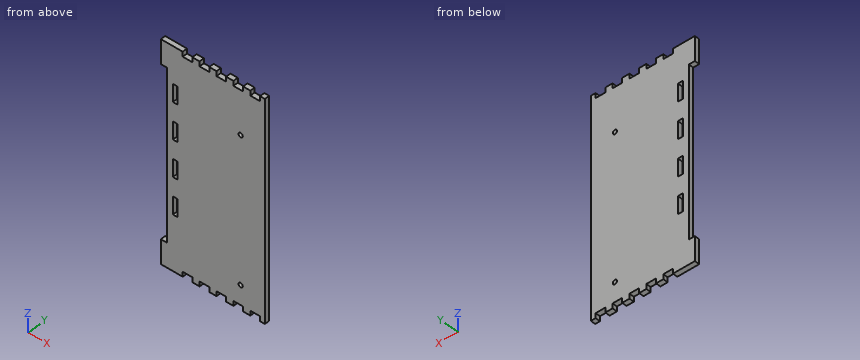
Autodesk Inventor part; units mm, degrees
ref_plane "YZ Plane" through (0, 0, 0) normal (1, 0, 0) x (0, 1, 0)
ref_plane "XZ Plane" through (0, 0, 0) normal (0, 1, 0) x (-1, 0, 0)
ref_plane "XY Plane" through (0, 0, 0) normal (0, 0, 1) x (1, 0, 0)
sketch "Sketch1" plane through (0, 0, 0) normal (0, 1, 0) x (-1, 0, 0)
  line L0 (-9.6671, 163.8128) -> (70.4329, 163.8128)
  line L1 (70.4329, 163.8128) -> (70.4329, -16.1872)
  line L2 (70.4329, -16.1872) -> (-9.6671, -16.1872)
  line L3 (-9.6671, -16.1872) -> (-9.6671, 163.8128)
  point P0 (0, 0)
extrude "Extrusion1" add sketch "Sketch1" along normal blind 4
sketch "Sketch2" plane through (0, 4, 0) normal (0, 1, 0) x (1, 0, 0)
  line L0 (-66.4329, -159.8128) -> (-66.4329, -148.8128)
  line L1 (-70.4329, -159.8128) -> (-70.4329, -148.8128)
  line L2 (-66.4329, -159.8128) -> (-66.4329, -148.8128)
  line L3 (-70.4329, -159.8128) -> (-70.4329, -148.8128)
  line L4 (-66.4329, -159.8128) -> (-66.4329, -148.8128)
  line L5 (-70.4329, -159.8128) -> (-70.4329, -148.8128)
  line L6 (-66.4329, -159.8128) -> (-66.4329, -148.8128)
  line L7 (-70.4329, -159.8128) -> (-70.4329, -148.8128)
  line L8 (-66.4329, -159.8128) -> (-66.4329, -148.8128)
  line L9 (-70.4329, -159.8128) -> (-70.4329, -148.8128)
  line L10 (-66.4329, -159.8128) -> (-66.4329, -148.8128)
  line L11 (-70.4329, -159.8128) -> (-70.4329, -148.8128)
  line L12 (-70.4329, -163.8128) -> (9.6671, -163.8128)
  line L13 (-30.3829, -163.8128) -> (-30.3829, 16.1872) construction
  line L14 (9.6671, 16.1872) -> (-70.4329, 16.1872)
  line L15 (-70.4329, -149.0628) -> (-66.4329, -149.0628)
  line L16 (-66.4329, -159.5628) -> (-70.4329, -159.5628)
  line L17 (-70.4329, 0.9372) -> (-66.4329, 0.9372)
  line L18 (-66.4329, -13.5628) -> (-70.4329, -13.5628)
  line L19 (-66.4329, -43.5628) -> (-70.4329, -43.5628)
  line L20 (-70.4329, -29.0628) -> (-66.4329, -29.0628)
  line L21 (-66.4329, -73.5628) -> (-70.4329, -73.5628)
  line L22 (-70.4329, -59.0628) -> (-66.4329, -59.0628)
  line L23 (-66.4329, -103.5628) -> (-70.4329, -103.5628)
  line L24 (-70.4329, -89.0628) -> (-66.4329, -89.0628)
  line L25 (-66.4329, -133.5628) -> (-70.4329, -133.5628)
  line L26 (-70.4329, -119.0628) -> (-66.4329, -119.0628)
  line L27 (5.6671, -159.8128) -> (5.6671, -148.8128)
  line L28 (9.6671, -159.8128) -> (9.6671, -148.8128)
  line L29 (5.6671, -133.8128) -> (5.6671, -118.8128)
  line L30 (9.6671, -133.8128) -> (9.6671, -118.8128)
  line L31 (5.6671, -103.8128) -> (5.6671, -88.8128)
  line L32 (9.6671, -103.8128) -> (9.6671, -88.8128)
  line L33 (5.6671, -73.8128) -> (5.6671, -58.8128)
  line L34 (9.6671, -73.8128) -> (9.6671, -58.8128)
  line L35 (5.6671, -43.8128) -> (5.6671, -28.8128)
  line L36 (9.6671, -43.8128) -> (9.6671, -28.8128)
  line L37 (5.6671, -13.8128) -> (5.6671, 1.1872)
  line L38 (9.6671, -13.8128) -> (9.6671, 1.1872)
  line L39 (9.6671, -149.0628) -> (5.6671, -149.0628)
  line L40 (5.6671, -159.5628) -> (9.6671, -159.5628)
  line L41 (9.6671, 0.9372) -> (5.6671, 0.9372)
  line L42 (5.6671, -13.5628) -> (9.6671, -13.5628)
  line L43 (5.6671, -43.5628) -> (9.6671, -43.5628)
  line L44 (9.6671, -29.0628) -> (5.6671, -29.0628)
  line L45 (5.6671, -73.5628) -> (9.6671, -73.5628)
  line L46 (9.6671, -59.0628) -> (5.6671, -59.0628)
  line L47 (5.6671, -103.5628) -> (9.6671, -103.5628)
  line L48 (9.6671, -89.0628) -> (5.6671, -89.0628)
  line L49 (5.6671, -133.5628) -> (9.6671, -133.5628)
  line L50 (9.6671, -119.0628) -> (5.6671, -119.0628)
  line L51 (-66.4329, -148.8128) -> (-70.4329, -148.8128)
  line L52 (-66.4329, -159.8128) -> (-70.4329, -159.8128)
  line L53 (-66.4329, -148.8128) -> (-70.4329, -148.8128)
  line L54 (-66.4329, -159.8128) -> (-70.4329, -159.8128)
  line L55 (-66.4329, -148.8128) -> (-70.4329, -148.8128)
  line L56 (-66.4329, -159.8128) -> (-70.4329, -159.8128)
  line L57 (-66.4329, -148.8128) -> (-70.4329, -148.8128)
  line L58 (-66.4329, -159.8128) -> (-70.4329, -159.8128)
  line L59 (-66.4329, -148.8128) -> (-70.4329, -148.8128)
  line L60 (-66.4329, -159.8128) -> (-70.4329, -159.8128)
  line L61 (-66.4329, -148.8128) -> (-70.4329, -148.8128)
  line L62 (-66.4329, -159.8128) -> (-70.4329, -159.8128)
  line L63 (-66.4329, -133.5628) -> (-66.4329, -119.0628)
  line L64 (-66.4329, -103.5628) -> (-66.4329, -89.0628)
  line L65 (-66.4329, -73.5628) -> (-66.4329, -59.0628)
  line L66 (-66.4329, -43.5628) -> (-66.4329, -29.0628)
  line L67 (-66.4329, -13.5628) -> (-66.4329, 0.9372)
  line L68 (-70.4329, 16.1872) -> (-70.4329, -163.8128)
  line L69 (9.6671, -163.8128) -> (9.6671, 16.1872)
  line L70 (1.6671, 16.1872) -> (1.6671, 12.1872)
  line L71 (1.6671, 12.1872) -> (-6.3329, 12.1872)
  line L72 (-6.3329, 12.1872) -> (-6.3329, 16.1872)
  line L73 (-12.3329, 16.1872) -> (-12.3329, 12.1872)
  line L74 (-12.3329, 12.1872) -> (-20.3329, 12.1872)
  line L75 (-20.3329, 12.1872) -> (-20.3329, 16.1872)
  line L76 (-26.3329, 16.1872) -> (-26.3329, 12.1872)
  line L77 (-26.3329, 12.1872) -> (-34.3329, 12.1872)
  line L78 (-34.3329, 12.1872) -> (-34.3329, 16.1872)
  line L79 (-40.3329, 16.1872) -> (-40.3329, 12.1872)
  line L80 (-40.3329, 12.1872) -> (-48.3329, 12.1872)
  line L81 (-48.3329, 12.1872) -> (-48.3329, 16.1872)
  line L82 (-54.3329, 16.1872) -> (-54.3329, 12.1872)
  line L83 (-54.3329, 12.1872) -> (-62.3329, 12.1872)
  line L84 (-62.3329, 12.1872) -> (-62.3329, 16.1872)
  line L85 (-12.3329, -73.8128) -> (-48.4329, -73.8128) construction
  line L86 (1.6671, -163.8128) -> (1.6671, -159.8128)
  line L87 (1.6671, -159.8128) -> (-6.3329, -159.8128)
  line L88 (-6.3329, -159.8128) -> (-6.3329, -163.8128)
  line L89 (-12.3329, -163.8128) -> (-12.3329, -159.8128)
  line L90 (-12.3329, -159.8128) -> (-20.3329, -159.8128)
  line L91 (-20.3329, -159.8128) -> (-20.3329, -163.8128)
  line L92 (-26.3329, -163.8128) -> (-26.3329, -159.8128)
  line L93 (-26.3329, -159.8128) -> (-34.3329, -159.8128)
  line L94 (-34.3329, -159.8128) -> (-34.3329, -163.8128)
  line L95 (-40.3329, -163.8128) -> (-40.3329, -159.8128)
  line L96 (-40.3329, -159.8128) -> (-48.3329, -159.8128)
  line L97 (-48.3329, -159.8128) -> (-48.3329, -163.8128)
  line L98 (-54.3329, -163.8128) -> (-54.3329, -159.8128)
  line L99 (-54.3329, -159.8128) -> (-62.3329, -159.8128)
  line L100 (-62.3329, -159.8128) -> (-62.3329, -163.8128)
  line L101 (9.6671, 1.1872) -> (5.6671, 1.1872)
  line L102 (9.6671, -13.8128) -> (5.6671, -13.8128)
  line L103 (9.6671, -28.8128) -> (5.6671, -28.8128)
  line L104 (9.6671, -43.8128) -> (5.6671, -43.8128)
  line L105 (9.6671, -58.8128) -> (5.6671, -58.8128)
  line L106 (5.6671, -73.8128) -> (9.6671, -73.8128)
  line L107 (9.6671, -88.8128) -> (5.6671, -88.8128)
  line L108 (9.6671, -103.8128) -> (5.6671, -103.8128)
  line L109 (9.6671, -118.8128) -> (5.6671, -118.8128)
  line L110 (9.6671, -133.8128) -> (5.6671, -133.8128)
  line L111 (9.6671, -148.8128) -> (5.6671, -148.8128)
  line L112 (9.6671, -159.8128) -> (5.6671, -159.8128)
  circle A0 centre (-14.3329, -3.8128) radius 1.75
  circle A1 centre (-14.3329, -123.8128) radius 1.75
  line L113 (5.6671, -163.8128) -> (5.6671, 16.1872)
  point P0 (0, 0)
  point P1 (-30.3829, -73.8128)
  point P2 (5.6671, 1.1872)
  dimension "d6" = 30
  dimension "d13" = 4
  dimension "d14" = 8
  dimension "d15" = 4
  dimension "d16" = 8
  dimension "d19" = 14
  dimension "d24" = 180
  dimension "d30" = 3.5
  dimension "d31" = 40
  dimension "d32" = 20
  dimension "d33" = 24
extrude "Extrusion2" cut sketch "Sketch2" against normal up to surface (4 mm away) contours L16 L1 L15 L0 | L100 L99 L98 L12 | L68 L26 L63 L25 | L97 L96 L95 L12 | L68 L24 L64 L23 | L94 L93 L92 L12 | L68 L22 L65 L21 | L91 L90 L89 L12 | L68 L20 L66 L19 | L88 L87 L86 L12 | L68 L17 L67 L18 | L113 L112 L69 L12 | L27 L40 L28 L112 | L27 L39 L28 L40 | L14 L82 L83 L84 | L27 L111 L28 L39 | L113 L110 L69 L111 | L14 L79 L80 L81 | L29 L49 L30 L110 | L29 L50 L30 L49 | L14 L76 L77 L78 | L29 L109 L30 L50 | L113 L108 L69 L109 | L14 L73 L74 L75 | L31 L47 L32 L108 | L31 L48 L32 L47 | L14 L70 L71 L72 | L31 L107 L32 L48 | L113 L106 L69 L107 | L14 L69 L101 L113 | L33 L45 L34 L106 | L101 L38 L41 L37 | L33 L46 L34 L45 | L41 L38 L42 L37 | L33 L105 L34 L46 | L42 L38 L102 L37 | L113 L104 L69 L105 | L102 L69 L103 L113 | L35 L43 L36 L104 | L103 L36 L44 L35 | L35 L44 L36 L43 | A0 | A1
sketch "Sketch4" plane through (0, 0, 0) normal (0, -1, 0) x (1, 0, 0)
  line L0 (-66.4329, 149.0628) -> (-70.4329, 149.0628)
  line L1 (-70.4329, 159.5628) -> (-70.4329, 163.8128)
  line L2 (-66.4329, 149.0628) -> (-70.4329, 149.0628)
  line L3 (-70.4329, 143.8128) -> (-70.4329, 159.5628)
  line L4 (-70.4329, 159.5628) -> (-66.4329, 159.5628)
  line L5 (-66.4329, 159.5628) -> (-66.4329, 149.0628)
  line L6 (-70.4329, 163.8128) -> (-80.4329, 163.8128)
  line L7 (-80.4329, 163.8128) -> (-80.4329, 143.8128)
  line L8 (-80.4329, 143.8128) -> (-70.4329, 143.8128)
  line L9 (-70.4329, 143.8128) -> (-70.4329, 163.8128)
  line L10 (-70.4329, -16.1872) -> (-70.4329, -0.9372)
  line L11 (-66.4329, 13.5628) -> (-70.4329, 13.5628)
  line L12 (-70.4329, 133.5628) -> (-70.4329, -0.9372)
  line L13 (-70.4329, -0.9372) -> (-66.4329, -0.9372)
  line L14 (-66.4329, -0.9372) -> (-66.4329, 13.5628)
  line L15 (-70.4329, 13.5628) -> (-66.4329, 13.5628)
  line L16 (-70.4329, -16.1872) -> (-80.4329, -16.1872)
  line L17 (-80.4329, -16.1872) -> (-80.4329, 3.8128)
  line L18 (-80.4329, 3.8128) -> (-70.4329, 3.8128)
  line L19 (-70.4329, 3.8128) -> (-70.4329, -16.1872)
  line L20 (-75.4329, 143.8128) -> (-75.4329, 3.8128)
  line L21 (-40.3329, 163.8128) -> (-40.3329, 159.8128)
  line L22 (-40.3329, 159.8128) -> (-48.3329, 159.8128)
  line L23 (-48.3329, 159.8128) -> (-48.3329, 163.8128)
  line L24 (-54.3329, 163.8128) -> (-48.3329, 163.8128)
  line L25 (-54.3329, 163.8128) -> (-54.3329, 159.8128)
  line L26 (-54.3329, 159.8128) -> (-62.3329, 159.8128)
  line L27 (-62.3329, 159.8128) -> (-62.3329, 163.8128)
  line L28 (-70.4329, 163.8128) -> (-62.3329, 163.8128)
  line L29 (-70.4329, 159.5628) -> (-70.4329, 163.8128)
  line L30 (-70.4329, 159.5628) -> (-66.4329, 159.5628)
  line L31 (-66.4329, 159.5628) -> (-66.4329, 149.0628)
  line L32 (-66.4329, 149.0628) -> (-70.4329, 149.0628)
  line L33 (-70.4329, 133.5628) -> (-70.4329, 149.0628)
  line L34 (-70.4329, 133.5628) -> (-66.4329, 133.5628)
  line L35 (-66.4329, 133.5628) -> (-66.4329, 119.0628)
  line L36 (-66.4329, 119.0628) -> (-70.4329, 119.0628)
  line L37 (-70.4329, 103.5628) -> (-70.4329, 119.0628)
  line L38 (-70.4329, 103.5628) -> (-66.4329, 103.5628)
  line L39 (-66.4329, 103.5628) -> (-66.4329, 89.0628)
  line L40 (-66.4329, 89.0628) -> (-70.4329, 89.0628)
  line L41 (-70.4329, 73.5628) -> (-70.4329, 89.0628)
  line L42 (-70.4329, 73.5628) -> (-66.4329, 73.5628)
  line L43 (-66.4329, 73.5628) -> (-66.4329, 59.0628)
  line L44 (-66.4329, 59.0628) -> (-70.4329, 59.0628)
  line L45 (-70.4329, 43.5628) -> (-70.4329, 59.0628)
  line L46 (-70.4329, 43.5628) -> (-66.4329, 43.5628)
  line L47 (-66.4329, 43.5628) -> (-66.4329, 29.0628)
  line L48 (-66.4329, 29.0628) -> (-70.4329, 29.0628)
  line L49 (-70.4329, 13.5628) -> (-70.4329, 29.0628)
  line L50 (-70.4329, 13.5628) -> (-66.4329, 13.5628)
  line L51 (-66.4329, 13.5628) -> (-66.4329, -0.9372)
  line L52 (-66.4329, -0.9372) -> (-70.4329, -0.9372)
  line L53 (-70.4329, -16.1872) -> (-70.4329, -0.9372)
  line L54 (-62.3329, -16.1872) -> (-70.4329, -16.1872)
  line L55 (-62.3329, -16.1872) -> (-62.3329, -12.1872)
  line L56 (-62.3329, -12.1872) -> (-54.3329, -12.1872)
  line L57 (-54.3329, -12.1872) -> (-54.3329, -16.1872)
  line L58 (-48.3329, -16.1872) -> (-54.3329, -16.1872)
  line L59 (-48.3329, -16.1872) -> (-48.3329, -12.1872)
  line L60 (-48.3329, -12.1872) -> (-40.3329, -12.1872)
  line L61 (-40.3329, -12.1872) -> (-40.3329, -16.1872)
  line L62 (-34.3329, -16.1872) -> (-40.3329, -16.1872)
  line L63 (-34.3329, -16.1872) -> (-34.3329, -12.1872)
  line L64 (-34.3329, -12.1872) -> (-26.3329, -12.1872)
  line L65 (-26.3329, -12.1872) -> (-26.3329, -16.1872)
  line L66 (-20.3329, -16.1872) -> (-26.3329, -16.1872)
  line L67 (-20.3329, -16.1872) -> (-20.3329, -12.1872)
  line L68 (-20.3329, -12.1872) -> (-12.3329, -12.1872)
  line L69 (-12.3329, -12.1872) -> (-12.3329, -16.1872)
  line L70 (-6.3329, -16.1872) -> (-12.3329, -16.1872)
  line L71 (-6.3329, -16.1872) -> (-6.3329, -12.1872)
  line L72 (-6.3329, -12.1872) -> (1.6671, -12.1872)
  line L73 (1.6671, -12.1872) -> (1.6671, -16.1872)
  line L74 (5.6671, -16.1872) -> (1.6671, -16.1872)
  line L75 (1.6671, 163.8128) -> (5.6671, 163.8128)
  line L76 (1.6671, 163.8128) -> (1.6671, 159.8128)
  line L77 (1.6671, 159.8128) -> (-6.3329, 159.8128)
  line L78 (-6.3329, 159.8128) -> (-6.3329, 163.8128)
  line L79 (-12.3329, 163.8128) -> (-6.3329, 163.8128)
  line L80 (-12.3329, 163.8128) -> (-12.3329, 159.8128)
  line L81 (-12.3329, 159.8128) -> (-20.3329, 159.8128)
  line L82 (-20.3329, 159.8128) -> (-20.3329, 163.8128)
  line L83 (-26.3329, 163.8128) -> (-20.3329, 163.8128)
  line L84 (-26.3329, 163.8128) -> (-26.3329, 159.8128)
  line L85 (-26.3329, 159.8128) -> (-34.3329, 159.8128)
  line L86 (-34.3329, 159.8128) -> (-34.3329, 163.8128)
  line L87 (-40.3329, 163.8128) -> (-34.3329, 163.8128)
  line L88 (5.6671, -16.1872) -> (5.6671, 163.8128)
  point P0 (0, 0)
  dimension "d25" = 10
  dimension "d26" = 20
  dimension "d29" = 5
extrude "Extrusion3" add sketch "Sketch4" against normal up to surface (4 mm away) contours L0 L3 L4 L5 | L3 L8 L7 L6 L1 | L33 L12 L18 L20 L8 | L18 L12 L10 L16 L17 | L12 L11 L14 L13
properties part number "side"
Work out the finished part from the listing and answer in its coordinate system (mm). Give positions to 0.01 mm unless a question says otherwise; leave off trailing zeros. Loops run counter-clockwise (first coordinate to the right, second up) from the corner with the lowest first, then second, coordinate; pieces in that order, holes last. Notation, with made-up numbers: (76.5, 78.25) -> (92.5, 78.25) arc R14 ccw to (92.5, 97.25) -> close; hole circle Ø5 at (41, -23). An arc over 180 degrees is marked (long way). Use a Markdown table: item, result. Add a question column.
1. Find the intervals of material crossed by probe 1 along Z at (x, y) = (-76, 2.75); probe 2 along X at (y, z) = (0.45, 36.5); probe 3 along X at (y, z) = (2, 137), in increasing order.
2. Section C-C on x = -32 is taken. Determine the outline of the cut face in (y, z), and give its area (3 significant figures).
3. Section B-B on z = 142 is taken. Determine the outline of the cut face in (x, y), and give its area (3 significant figures).
4. Flat-ended cylindrical pins translate along their axes: pin 1 Ø2 at (y, z) = (1.5, 128) entering from -X; pin 2 Ø1.5 at (x, z) = (-63, 21) entering from -Y; pin 3 Ø2 at (x, y) = (-44.5, 3) entering from -Z. Find the tip coordinate at first contact, or state that the pin passes through.
5. Section A-A on x = -68.5 is taken. Determine the outline of the cut face in (y, z), and give its area (3 significant figures).
6. Section D-D on y = 3.05 is taken. State how many separate pieces and enclosed holes the cut face has, and give its area (3 significant figures).
Results below:
| question | item | result |
|---|---|---|
| 1 | probe 1 | z = -16.19 to 3.81, 143.81 to 163.81 |
| 1 | probe 2 | x = -75.43 to -70.43, -66.43 to 5.67 |
| 1 | probe 3 | x = -75.43 to 5.67 |
| 2 | outline | (0, -12.19) -> (4, -12.19) -> (4, 159.81) -> (0, 159.81) -> close |
| 2 | area | 688 mm^2 |
| 3 | outline | (-75.43, 0) -> (5.67, 0) -> (5.67, 4) -> (-75.43, 4) -> close |
| 3 | area | 324 mm^2 |
| 4 | pin 1 | stops at x = -75.43 |
| 4 | pin 2 | stops at y = 0 |
| 4 | pin 3 | stops at z = -12.19 |
| 5 | outline | (0, -16.19) -> (4, -16.19) -> (4, 29.06) -> (0, 29.06) -> close; (0, 43.56) -> (4, 43.56) -> (4, 59.06) -> (0, 59.06) -> close; (0, 73.56) -> (4, 73.56) -> (4, 89.06) -> (0, 89.06) -> close; (0, 103.56) -> (4, 103.56) -> (4, 119.06) -> (0, 119.06) -> close; (0, 133.56) -> (4, 133.56) -> (4, 163.81) -> (0, 163.81) -> close |
| 5 | area | 488 mm^2 |
| 6 | separate pieces | 1 |
| 6 | enclosed holes | 6 |
| 6 | area | 14,200 mm^2 |
